Autodesk Inventor part; units mm, degrees
ref_plane "YZ Plane" through (0, 0, 0) normal (1, 0, 0) x (0, 1, 0)
ref_plane "XZ Plane" through (0, 0, 0) normal (0, 1, 0) x (-1, 0, 0)
ref_plane "XY Plane" through (0, 0, 0) normal (0, 0, 1) x (1, 0, 0)
sketch "Sketch1" plane through (0, 0, 0) normal (0, 0, 1) x (1, 0, 0)
  line L0 (-104.14, 12.7) -> (104.14, 12.7)
  line L1 (104.14, 12.7) -> (104.14, -12.7)
  line L2 (104.14, -12.7) -> (-104.14, -12.7)
  line L3 (-104.14, -12.7) -> (-104.14, 12.7)
  line L4 (-104.14, 12.7) -> (104.14, -12.7) construction
  line L5 (104.14, 12.7) -> (-104.14, -12.7) construction
  point P0 (0, 0)
  dimension "d0" = 208.28
  dimension "d1" = 25.4
extrude "Extrusion1" add sketch "Sketch1" along normal mid plane 50.8
sketch "Sketch2" plane through (0, 0, 25.4) normal (0, 0, 1) x (1, 0, 0)
  line L0 (-104.14, 12.7) -> (-104.14, -12.7)
  line L1 (-104.14, -12.7) -> (104.14, -12.7)
  point P0 (0, 0)
  point P1 (0, 13.4938)
  dimension "d5" = 104.14
  dimension "d13" = 26.1938
hole "Hole1" at (0, 13.4938, 25.4) direction (0, 0, -1) diameter 38.1 end through all
sketch "Sketch3" plane through (0, 0, 25.4) normal (0, 0, 1) x (1, 0, 0)
  line L0 (-6.35, 12.7) -> (6.35, 12.7)
  line L1 (6.35, 12.7) -> (6.35, -6.35)
  line L2 (6.35, -6.35) -> (-6.35, -6.35)
  line L3 (-6.35, -6.35) -> (-6.35, 12.7)
  line L4 (104.14, 12.7) -> (19.0335, 12.7)
  line L5 (-104.14, 12.7) -> (-104.14, -12.7)
  point P0 (0, 0)
  dimension "d14" = 19.05
  dimension "d15" = 19.05
  dimension "d16" = 12.7
  dimension "d17" = 97.79
extrude "Extrusion2" cut sketch "Sketch3" against normal through all
equation "\"d0\" = kn_wid"
equation "\"d1\" = kn_hei"
equation "\"d2\" = kn_len"
equation "\"d6\" = kn_hole_diam"
equation "\"d14\" = kn_groove_hei"
equation "\"d15\" = kn_groove_hei"
equation "\"d16\" = kn_groove_wid"
equation "\"d17\" = 0.5 * kn_wid - 0.5 * kn_groove_wid"
properties part number "kfnmount" material "Aluminum 6061"
The listing builds one solid part. Answer for the finished solid, in the listing's coordinates (mm). A direction names the side the tool comes from. Give positions to 0.01 mm unless a question says otherwise; leave off trailing zeros. Write each loop counter-clockwise with the first axis right and the second up, starting at its lowest first coordinate (ties: lowest second). Pieces come first, ordered by that corner, then holes.
1) Find the intervals of material crossed by L1, parallel to X at y = -4.5, z = -22; L2, parallel to X at y = 0.25, z = 4.5; L3, parallel to Y at x = -3, z = 20.5, in increasing order.
2) Section C-C (x = 4.5) is taken. Write down the section's boundary in (y, z).
3) Section B-B (z = -22) is taken. Write down the section's boundary in (x, y).
4) For a pull along X with two mould halves and no side action, classify faces 3 (the face through (-15.23, 2.05, -0.36)), 4 (the face through (0, -6.35, 0)), 5 (the face through (61, 12.7, 0)), 6 (the face through (-104.14, 0, 0)) as pulls with the +X half, pulls with the -X half, needs draft (parallel to the pull), parting line crosses it, or undercut.
5) Section A-A (y = 9.5) is taken. Write down the section's boundary in (x, z).
6) A tool of negligible diameter and unlimited length cuts with its end or side. For faces 1 (the face through (15.415, 2.301, -0.356)), 2 (the face through (104.14, 0, 0)), from which of +Z, -Z, +X, -X, +Y, -Y can it reach the whole face along a straight path? Write none if from no direction.
7) Given P1, Ø14, axis at x = 0.5, z = -1, coming from the +Y side, flat-ended and moving along its own axis, determine where the tip first touches the part or whether it passes through.
Response:
1. L1: x = -104.14 to -6.35, 6.35 to 104.14
1. L2: x = -104.14 to -13.69, 13.69 to 104.14
1. L3: y = -12.7 to -6.35
2. outline: (-12.7, -25.4) - (-6.35, -25.4) - (-6.35, 25.4) - (-12.7, 25.4) - close
3. outline: (-104.14, -12.7) - (104.14, -12.7) - (104.14, 12.7) - (19.03, 12.7) arc R19.05 cw to (6.35, -4.47) - (6.35, -6.35) - (-6.35, -6.35) - (-6.35, -4.47) arc R19.05 cw to (-19.03, 12.7) - (-104.14, 12.7) - close
4. face 3: undercut
4. face 4: undercut
4. face 5: needs draft
4. face 6: pulls with the -X half
5. outline: (-104.14, -25.4) - (-18.63, -25.4) - (-18.63, 25.4) - (-104.14, 25.4) - close; (18.63, -25.4) - (104.14, -25.4) - (104.14, 25.4) - (18.63, 25.4) - close
6. face 1: +Z, -Z, +Y
6. face 2: +Z, -Z, +X, +Y, -Y
7. P1: stops at y = -4.02
